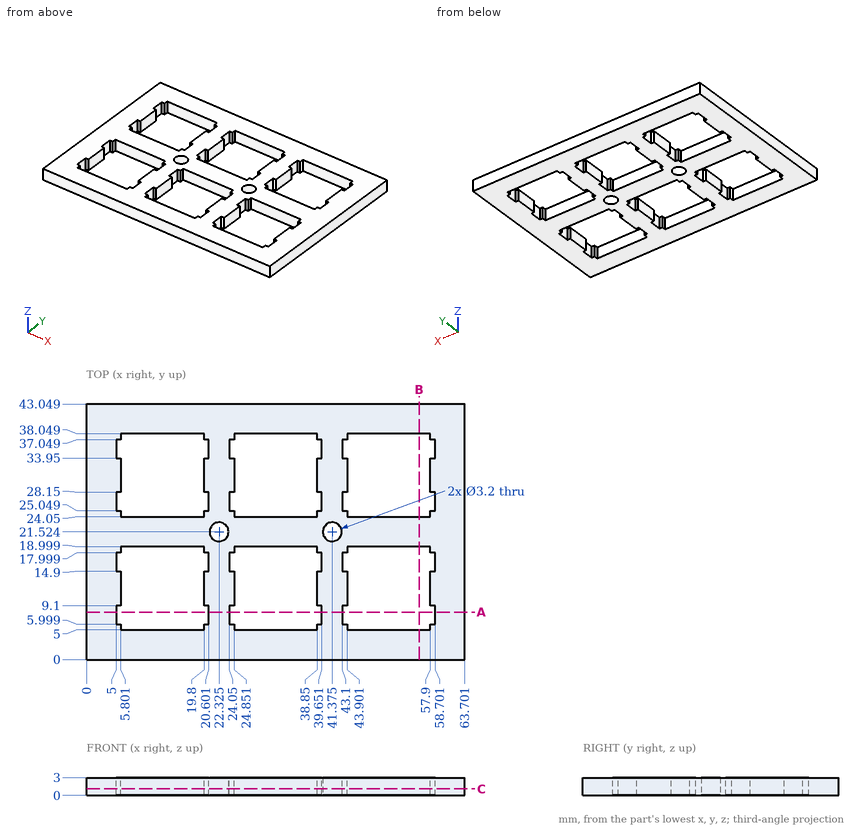
Here's the drawing with two shaded views (mm, measured from the low corner). I have some questions. Coordinates: 2 decimals unless noted, no trailing zeros. Loops run counter-clockwise (first coordinate to the right, second up) from the corner with the lowest first, then second, coordinate; pieces in that order, holes last. Notation, with made-up numbers: M 39.5,-35.75 L 87.5,-35.75 A23 ccw 87.5,-16.75 Z; hole C -7,25 d11. An arc over 180 degrees is marked long. Put each result on its own line as item: value. Start each with the question number.
(1) I need wall thicknesses on probe 1 along Y at (x, z) = (15.5, 1.45); probe 2 along X at (y, z) = (35, 2.55); probe 3 along X at (y, z) = (29.5, 1.75). Which ranges of each line are inside material? Lowest first, please.
(2) Imagine slicing it at C-C on z = 1.1. Give the number of separate pieces and of enclosed holes in the cut face, and give its area (3 significant figures).
(3) Imagine slicing it at A-A on y = 8. List the corners of the cut face in (x, z) for me.
(4) Imagine slicing it at B-B on x = 56. List the corners of the cut face in (y, z) for me.
Worked answers:
1. probe 1: y = 0 to 5, 19 to 24.05, 38.05 to 43.05
1. probe 2: x = 0 to 5, 20.6 to 24.05, 39.65 to 43.1, 58.7 to 63.7
1. probe 3: x = 0 to 5.8, 19.8 to 24.85, 38.85 to 43.9, 57.9 to 63.7
2. separate pieces: 1
2. enclosed holes: 8
2. area: 1,490 mm2
3. outline: M 0,0 L 5,0 L 5,3 L 0,3 Z; M 20.6,0 L 24.05,0 L 24.05,3 L 20.6,3 Z; M 39.65,0 L 43.1,0 L 43.1,3 L 39.65,3 Z; M 58.7,0 L 63.7,0 L 63.7,3 L 58.7,3 Z
4. outline: M 0,0 L 5,0 L 5,3 L 0,3 Z; M 19,0 L 24.05,0 L 24.05,3 L 19,3 Z; M 38.05,0 L 43.05,0 L 43.05,3 L 38.05,3 Z
